from build123d import *

# Parameters (mm, degrees)
SKETCH1_W           = 115.062
SKETCH1_H           = 214.884
BOSS_EXTRUDE1_DEPTH = 50.038
SKETCH2_W           = 113.4745
SKETCH2_H           = 12.7
CUT_EXTRUDE1_DEPTH  = 48.4505
FILLET2_R           = 1.5875
SHELL2_START        = 1.5875
SHELL2_OUTLINE_W    = 111.887
SHELL2_OUTLINE_H    = 199.009
SHELL2_DEPTH        = 46.863
SHELL2_2_OUTLINE_W  = 98.886987896
SHELL2_2_OUTLINE_H  = 1.5875
SHELL2_2_DEPTH      = 29.689064402
SKETCH3_W           = 98.886987896
SKETCH3_H           = 64.932506417
BOSS_EXTRUDE2_DEPTH = 17.8435
CUT_EXTRUDE2_REACH  = 227.021
SKETCH5_W           = 6.35
SKETCH5_H           = 4.550671723
LPATTERN1_COUNT     = 12
LPATTERN1_PITCH     = 7.9375


# Read off the part's stored shape, not the designer's step: Shell2
with BuildPart() as part:
    # Sketch1 → Boss-Extrude1 (new body)
    with BuildSketch(Plane(origin=(0, 0, 0), x_dir=(1, 0, 0), z_dir=(0, 1, 0))):
        Rectangle(SKETCH1_W, SKETCH1_H)
    extrude(amount=BOSS_EXTRUDE1_DEPTH)

    # Sketch2 → Cut-Extrude1 (cut)
    with BuildSketch(Plane(origin=(0, 50.038, 0), x_dir=(1, 0, 0), z_dir=(0, 1, 0))):
        with Locations((-0.79375, -101.092)):
            Rectangle(SKETCH2_W, SKETCH2_H)
    extrude(amount=-CUT_EXTRUDE1_DEPTH, mode=Mode.SUBTRACT)

    # Fillet2
    fillet2_edges = [part.edges().sort_by_distance(p)[0] for p in [
        (-57.531, 0, 0),
        (-57.531, 50.038, -6.35),
        (57.531, 0, 0),
        (57.531, 50.038, 0),
    ]]
    fillet(fillet2_edges, radius=FILLET2_R)

    # Shell2 outline → Shell2 (cut)
    with BuildSketch(Plane(origin=(0, 0, 0), x_dir=(1, 0, 0), z_dir=(0, 1, 0)).offset(SHELL2_START)):
        with Locations((0, 6.35)):
            Rectangle(SHELL2_OUTLINE_W, SHELL2_OUTLINE_H)
    extrude(amount=SHELL2_DEPTH, mode=Mode.SUBTRACT)

    # Shell2 2 outline → Shell2 2 (cut)
    with BuildSketch(Plane(origin=(0, 0, 0), x_dir=(1, 0, 0), z_dir=(0, 1, 0)).offset(SHELL2_START)):
        with Locations((6.500006052, -93.94825)):
            Rectangle(SHELL2_2_OUTLINE_W, SHELL2_2_OUTLINE_H)
    extrude(amount=SHELL2_2_DEPTH, mode=Mode.SUBTRACT)

    # Sketch3 → Boss-Extrude2 (add)
    with BuildSketch(Plane(origin=(0, 1.5875, 0), x_dir=(1, 0, 0), z_dir=(0, 1, 0))):
        with Locations((6.500006052, -71.800746792)):
            Rectangle(SKETCH3_W, SKETCH3_H)
    extrude(amount=BOSS_EXTRUDE2_DEPTH)

    # Sketch5 → Cut-Extrude2 (cut, up to next)
    with BuildSketch(Plane.XY.offset(104.267), mode=Mode.PRIVATE) as cut_extrude2_sk1:
        with Locations((51.181, 17.155664139)):
            Rectangle(SKETCH5_W, SKETCH5_H)
    cut_extrude2_tool1 = extrude(cut_extrude2_sk1.sketch, amount=-CUT_EXTRUDE2_REACH, mode=Mode.PRIVATE) & part.part
    cut_extrude2 = cut_extrude2_tool1.solids().sort_by_distance((51.181, 17.155664, 104.267))[0]
    add(cut_extrude2, mode=Mode.SUBTRACT)

    # LPattern1: Cut-Extrude2 ×12
    with Locations(*[(-i * LPATTERN1_PITCH, 0, 0) for i in range(1, LPATTERN1_COUNT)]):
        add(cut_extrude2, mode=Mode.SUBTRACT)


solid = part.part
The model under review builds one solid part; all positions refer to its coordinate system, in mm. A direction names the side the tool comes from. Round coordinates to 2 decimals unless told otherwise and drop trailing zeros. Write each loop counter-clockwise with the first axis right and the second up, starting at its lowest first coordinate (ties: lowest second). Pieces come first, ordered by that corner, then holes. Notation, with made-up numbers: (-32, -3) -> (10, -3) arc R26 ccw to (10, 19) -> close; hole circle Ø7 at (83, -16.5). An arc over 180 degrees is marked (long way). Answer as a JSON object with one key per item and string values.
1. We need section B-B on x = 42.5. State the section outline as (y, z) points.
Results found:
{"outline": "(0, -107.44) -> (50.04, -107.44) -> (50.04, 94.74) -> (31.28, 94.74) -> (31.28, 93.15) -> (48.45, 93.15) -> (48.45, -105.85) -> (1.59, -105.85) -> (1.59, 39.33) -> (14.88, 39.33) -> (14.88, 104.27) -> (1.59, 104.27) -> (1.59, 107.44) -> (0, 107.44) -> close"}
2. Clearance check with flat-ended pins moving along their axes: pin 1 (6.5 mm diameter, centred on x = -17, z = 99, fed in from +Y); pin 2 (2 mm diameter, centred on x = 2.5, y = 8.5, fed in from +Z). State where each tip first meets the part, or that it passes through.
Results found:
{"pin 1": "stops at y = 19.43", "pin 2": "stops at z = 104.27"}
3. We need section D-D on y = 28.5. State the section outline as (x, z) points.
Results found:
{"outline": "(-57.53, -107.44) -> (57.53, -107.44) -> (57.53, 107.44) -> (55.94, 107.44) -> (55.94, -105.85) -> (-55.94, -105.85) -> (-55.94, 93.15) -> (-42.94, 93.15) -> (-42.94, 94.74) -> (-57.53, 94.74) -> close"}
4. Machinability: for faces 3 (the face through (-1, 1.587, -30)), 4 (the face through (32.131, 17, 72)), which of the approach directions +Z, -Z, +X, -X, +Y, -Y give a long, thin tool a straight path to every point of the face, cutting with its end or side? Answer none if there is none.
Results found:
{"face 3": "none", "face 4": "+Z"}
5. We need section A-A on z = 33. State the section outline as (x, y) points (1 decimal), and give its area (3 significant figures).
Results found:
{"outline": "(-57.5, 1.6) arc R1.6 ccw to (-55.9, 0) -> (55.9, 0) arc R1.6 ccw to (57.5, 1.6) -> (57.5, 48.5) arc R1.6 ccw to (55.9, 50) -> (-55.9, 50) arc R1.6 ccw to (-57.5, 48.5) -> close; hole (-55.9, 1.6) -> (55.9, 1.6) -> (55.9, 48.5) -> (-55.9, 48.5) -> close", "area": "512 mm^2"}
6. To check wall thickness, follow line 1 along X through (y, z) = (28, -80.5); line 2 along Y through (x, z) = (-20, 13.5); line 3 along Z through (x, y) = (18, 35.5). State the ranges of each line that lie inside material, in increasing order.
Results found:
{"line 1": "x = -57.53 to -55.94, 55.94 to 57.53", "line 2": "y = 0 to 1.59, 48.45 to 50.04", "line 3": "z = -107.44 to -105.85, 93.15 to 94.74"}
7. The part is to be moulded in two halves that separate along Y. For faces 1 (the face through (6, 8, 104.267)), 2 (the face through (30.543, 17, 72)), say which applies: pulls with the +Y half, pulls with the -Y half, needs draft (parallel to the pull), parting line crosses it, or undercut.
Results found:
{"face 1": "needs draft", "face 2": "undercut"}
8. We need section C-C on y = 4. State the section outline as (x, z) points, and give its area (3 significant figures).
Results found:
{"outline": "(-57.53, -107.44) -> (57.53, -107.44) -> (57.53, 107.44) -> (55.94, 107.44) -> (55.94, 104.27) -> (-42.94, 104.27) -> (-42.94, 94.74) -> (-57.53, 94.74) -> close; hole (-55.94, -105.85) -> (55.94, -105.85) -> (55.94, 39.33) -> (-42.94, 39.33) -> (-42.94, 93.15) -> (-55.94, 93.15) -> close", "area": "7,280 mm^2"}
